Can you work these out from the drawing? Everything is in mm from the part's minimum corner. Round coordinates to 2 decimals unless told otherwise and drop trailing zeros. Order: outer loops, then holes, each group sorted by start corner. A loop starts at its lowest first (then second) coordinate and runs counter-clockwise, first axis right, second up. Notation, with made-up numbers: M 2.25,-10.5 L 57.25,-10.5 A24 cw 57.25,23.5 Z; hole C 61,70 d6. An arc over 180 degrees is marked long. Answer as a JSON object with one key per item and string values. Group by question number.
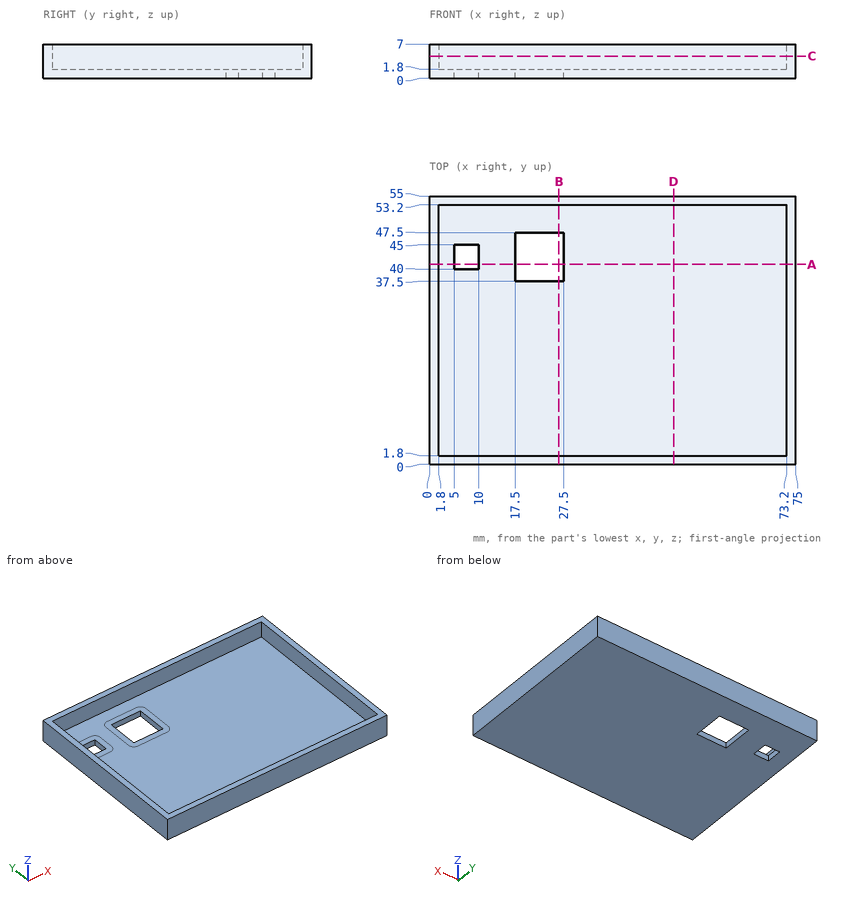
Item 1: Suppose I cut it at D-D, the plane x = 50. Write out the boundary of the cut face in (y, z).
Item 2: I'm going to push a flat-ended pin straight in: pin 1 Ø2.5 at (x, y) = (7, 44) entering from +Z. Where does the tip first touch, or does it pass through?
Item 3: Suppose I cut it at A-A, the plane y = 41. Write out the boundary of the cut face in (x, z), and give its area (3 significant figures).
Item 4: Suppose I cut it at C-C, the plane z = 4.5. Write out the boundary of the cut face in (x, y), and give its area (3 significant figures).
Item 5: Suppose I cut it at B-B, the plane x = 26.5. Write out the boundary of the cut face in (y, z), and give its area (3 significant figures).
Item 6: I need wall thicknesses on line 1 (X direction, y = 42.5, z = 1.5); line 2 (X direction, y = 25, z = 2); line 3 (Y direction, x = 24.5, z = 2.5). Which ranges of each line are inside material? Lowest first, please.
Computed:
{
 "1": {"outline": "M 0,0 L 55,0 L 55,7 L 53.2,7 L 53.2,1.8 L 1.8,1.8 L 1.8,7 L 0,7 Z"},
 "2": {"pin 1": "stops at z = 1.8"},
 "3": {"outline": "M 0,0 L 5,0 L 5,1.8 L 1.8,1.8 L 1.8,7 L 0,7 Z; M 10,0 L 17.5,0 L 17.5,1.8 L 10,1.8 Z; M 27.5,0 L 75,0 L 75,7 L 73.2,7 L 73.2,1.8 L 27.5,1.8 Z", "area": "127 mm^2"},
 "4": {"outline": "M 0,0 L 75,0 L 75,55 L 0,55 Z; hole M 1.8,1.8 L 73.2,1.8 L 73.2,53.2 L 1.8,53.2 Z", "area": "455 mm^2"},
 "5": {"outline": "M 0,0 L 37.5,0 L 37.5,1.8 L 1.8,1.8 L 1.8,7 L 0,7 Z; M 47.5,0 L 55,0 L 55,7 L 53.2,7 L 53.2,1.8 L 47.5,1.8 Z", "area": "99.7 mm^2"},
 "6": {"line 1": "x = 0 to 5, 10 to 17.5, 27.5 to 75", "line 2": "x = 0 to 1.8, 73.2 to 75", "line 3": "y = 0 to 1.8, 53.2 to 55"}
}
